Autodesk Inventor part; units mm, degrees
ref_plane "YZ Plane" through (0, 0, 0) normal (1, 0, 0) x (0, 1, 0)
ref_plane "XZ Plane" through (0, 0, 0) normal (0, 1, 0) x (-1, 0, 0)
ref_plane "XY Plane" through (0, 0, 0) normal (0, 0, 1) x (1, 0, 0)
sketch "Skizze1" plane through (0, 0, 0) normal (0, 0, 1) x (1, 0, 0)
  line L0 (-110, -110) -> (110, -110)
  line L1 (110, -110) -> (110, 110)
  line L2 (110, 110) -> (-110, 110)
  line L3 (-110, 110) -> (-110, -110)
  line L4 (-110, -110) -> (110, 110) construction
  line L5 (110, -110) -> (-110, 110) construction
  circle A0 centre (0, 0) radius 95 construction
  circle A1 centre (0, 0) radius 105 construction
  line L6 (-90, 90) -> (-110, 90) construction
  line L7 (-110, 90) -> (-110, 110) construction
  line L8 (-110, 110) -> (-90, 110) construction
  line L9 (-90, 110) -> (-90, 90) construction
  line L10 (-90, 90) -> (-110, 110) construction
  line L11 (-110, 90) -> (-90, 110) construction
  line L12 (110, -110) -> (-110, -110)
  line L13 (-110, -110) -> (-110, -180)
  line L14 (-110, -180) -> (110, -180)
  line L15 (110, -180) -> (110, -110)
  line L16 (90, 90) -> (110, 90) construction
  line L17 (110, 90) -> (110, 110) construction
  line L18 (110, 110) -> (90, 110) construction
  line L19 (90, 110) -> (90, 90) construction
  line L20 (90, 90) -> (110, 110) construction
  line L21 (110, 90) -> (90, 110) construction
  line L22 (90, -160) -> (110, -160) construction
  line L23 (110, -160) -> (110, -180) construction
  line L24 (110, -180) -> (90, -180) construction
  line L25 (90, -180) -> (90, -160) construction
  line L26 (90, -160) -> (110, -180) construction
  line L27 (110, -160) -> (90, -180) construction
  line L28 (-90, -160) -> (-110, -160) construction
  line L29 (-110, -160) -> (-110, -180) construction
  line L30 (-110, -180) -> (-90, -180) construction
  line L31 (-90, -180) -> (-90, -160) construction
  line L32 (-90, -160) -> (-110, -180) construction
  line L33 (-110, -160) -> (-90, -180) construction
  line L34 (-90, -90) -> (-110, -90) construction
  line L35 (-110, -90) -> (-110, -110) construction
  line L36 (-110, -110) -> (-90, -110) construction
  line L37 (-90, -110) -> (-90, -90) construction
  line L38 (-90, -90) -> (-110, -110) construction
  line L39 (-110, -90) -> (-90, -110) construction
  line L40 (90, -90) -> (110, -90) construction
  line L41 (110, -90) -> (110, -110) construction
  line L42 (110, -110) -> (90, -110) construction
  line L43 (90, -110) -> (90, -90) construction
  line L44 (90, -90) -> (110, -110) construction
  line L45 (110, -90) -> (90, -110) construction
  circle A2 centre (0, 0) radius 87.5
  line L46 (110, 45.5635) -> (45.5635, 110) construction
  line L47 (-45.5635, 110) -> (-110, 45.5635) construction
  line L48 (45.5635, 110) -> (-45.5635, 110)
  line L49 (-45.5635, 110) -> (45.5635, 110) construction
  line L50 (45.5635, 110) -> (110, 45.5635) construction
  line L51 (110, 45.5635) -> (110, -45.5635) construction
  line L52 (110, -45.5635) -> (45.5635, -110) construction
  line L53 (45.5635, -110) -> (-45.5635, -110) construction
  line L54 (-45.5635, -110) -> (-110, -45.5635) construction
  line L55 (-110, -45.5635) -> (-110, 45.5635) construction
  line L56 (-110, 45.5635) -> (-45.5635, 110) construction
  line L57 (110, 0) -> (110, 110)
  line L58 (-110, 0) -> (-110, 110)
  line L59 (110, 0) -> (110, 110)
  line L60 (110, 110) -> (-110, 110)
  line L61 (-110, 110) -> (-110, 0)
  arc A3 (110, 0) -> (0, 110) centre (0, 0) ccw
  arc A4 (0, 110) -> (-110, 0) centre (0, 0) ccw
  circle A5 centre (100, -170) radius 18.5 construction
  circle A6 centre (100, -35) radius 18.5 construction
  circle A7 centre (70.7107, 70.7107) radius 18.5 construction
  circle A8 centre (-70.7107, 70.7107) radius 18.5 construction
  circle A9 centre (-100, -35) radius 18.5 construction
  circle A10 centre (0, 0) radius 100 construction
  line L62 (100, -170) -> (100, 100) construction
  line L63 (-100, -170) -> (-100, 100) construction
  line L64 (110, -20) -> (110, 0) construction
  line L65 (110, 0) -> (90, -70) construction
  line L66 (-110, -20) -> (-110, 0) construction
  point P0 (-100, -100)
  point P1 (100, -100)
  dimension "d0" = 190
  dimension "d1" = 10
  dimension "d2" = 220
  dimension "d3" = 20
  dimension "d4" = 70
  dimension "d14" = 175
  dimension "d15" = 45
  dimension "d16" = 45
  dimension "d21" = 37
  dimension "d25" = 10
  dimension "d26" = 145
  dimension "d27" = 145
  dimension "d28" = 10
  dimension "d29" = 200
extrude "Extrusion1" add sketch "Skizze1" along normal blind 5 contours L3 A4 A3 L1 L0 | L0 L15 L14 L13 | L3 L2 A4 | A3 L2 L1 | A2
hole "Bohrung1" at (100, -170, 0) at (-100, -170, 0) at (-100, 100, 0) at (100, 100, 0) at (-100, -35, 0) at (-70.7107, 70.7107, 0) at (70.7107, 70.7107, 0) at (100, -35, 0) direction (0, 0, 1) diameter 5.3 end through all
sketch "Skizze2" plane through (0, 0, 5) normal (0, 0, 1) x (1, 0, 0)
  circle A0 centre (-100, 100) radius 2.65
  circle A1 centre (100, -170) radius 2.65
  circle A2 centre (-100, -170) radius 2.65
  circle A3 centre (100, 100) radius 2.65
  line L0 (-110, 110) -> (-110, -180)
  line L1 (-110, -180) -> (110, -180)
  line L2 (110, -180) -> (110, 110)
  line L3 (110, 110) -> (-110, 110)
  arc A4 (110, 0) -> (-110, 0) centre (0, 0) ccw
  line L4 (110, -180) -> (110, 110)
  line L5 (-110, 110) -> (-110, -180)
  line L6 (110, 110) -> (-110, 110)
  dimension "d22" = 50
  dimension "d23" = 35
extrude "Extrusion3" cut sketch "Skizze2" against normal through all contours L3 A4 L0 | L3 L2 A4
ref_plane "Arbeitsebene1" through (0, -180, 0) normal (-1, 0, 0) x (0, 0, 1)
equation "\"d16\" = d15"
properties part number "BasePlate_A" material "Aluminium 6061"
The listing builds one solid part. Answer for the finished solid, in the listing's coordinates (mm). Coordinates: 2 decimals unless noted, no trailing zeros. Loops run counter-clockwise (first coordinate to the right, second up) from the corner with the lowest first, then second, coordinate; pieces in that order, holes last. Notation, with made-up numbers: (17.25, 77.25) - (30.25, 77.25) arc R25 cw to (30.25, 101.25) - close; hole circle Ø1 at (43.5, 27.25). An arc over 180 degrees is marked (long way). Use a Markdown table: item, result. Add a question column.
1) The part is cut by section C-C, the plane x = 35. Give the vertices of the cut face in (y, z), and give its area (3 significant figures).
2) The part is cut by section A-A, the plane z = 4. Give the vertices of the cut face in (x, y), and give its area (3 significant figures).
3) Find the intervals of material crossed by line 1 (X direction, y = -35, z = 2.2); line 2 (Y direction, x = 99, z = 0.8); line 3 (Y direction, x = 100, z = 2.55), in increasing order.
4) The mould has two halves that part along Z. Classify faces 1 (the cylindrical face through (2.419, 109.973, 2.535)), 2 (the flat face through (-2, -33, 0)), 3 (the flat face through (-2, -33, 5)): released by +Z, released by -Z, zero draft, split by the parting line, or undercut.
5) The part is cut by section B-B, the plane x = -87.5. Give the vertices of the cut face in (y, z), and give its area (3 significant figures).
Here are the results:
| question | item | result |
|---|---|---|
| 1 | outline | (-180, 0) - (104.28, 0) - (104.28, 5) - (-180, 5) - close |
| 1 | area | 1,420 mm^2 |
| 2 | outline | (-110, -180) - (110, -180) - (110, 0) arc R110 ccw to (-110, 0) - close; hole circle Ø5.3 at (-100, -170); hole circle Ø5.3 at (-100, -35); hole circle Ø5.3 at (-70.71, 70.71); hole circle Ø5.3 at (70.71, 70.71); hole circle Ø5.3 at (100, -170); hole circle Ø5.3 at (100, -35) |
| 2 | area | 58,500 mm^2 |
| 3 | line 1 | x = -110 to -102.65, -97.35 to 97.35, 102.65 to 110 |
| 3 | line 2 | y = -180 to -172.45, -167.55 to -37.45, -32.55 to 47.95 |
| 3 | line 3 | y = -180 to -172.65, -167.35 to -37.65, -32.35 to 45.83 |
| 4 | face 1 | zero draft |
| 4 | face 2 | released by -Z |
| 4 | face 3 | released by +Z |
| 5 | outline | (-180, 0) - (66.66, 0) - (66.66, 5) - (-180, 5) - close |
| 5 | area | 1,230 mm^2 |
